```python
from build123d import *

# Parameters (mm, degrees)
SKETCH1_R           = 13.97
SKETCH1_R_2         = 1.651
BOSS_EXTRUDE1_DEPTH = 4.7625
LEG1_DEPTH          = 4.826
FILLET2_R           = 10


with BuildPart() as part:
    # Sketch1 → Boss-Extrude1 (new body)
    with BuildSketch(Plane(origin=(0, 0, 0), x_dir=(0, 0, -1), z_dir=(1, 0, 0))):
        with Locations(Location((0, 0, 0), (0, 0, 180))):
            Circle(SKETCH1_R)
        with Locations(Location((-10.16, 0, 0), (0, 0, 180))):
            Circle(SKETCH1_R_2, mode=Mode.SUBTRACT)
        with Locations(Location((0, 10.16, 0), (0, 0, 180))):
            Circle(SKETCH1_R_2, mode=Mode.SUBTRACT)
        with Locations(Location((10.16, 0, 0), (0, 0, 180))):
            Circle(SKETCH1_R_2, mode=Mode.SUBTRACT)
        with Locations(Location((0, -10.16, 0), (0, 0, 180))):
            Circle(SKETCH1_R_2, mode=Mode.SUBTRACT)
    extrude(amount=BOSS_EXTRUDE1_DEPTH)

    # Sketch2 → leg1 (add)
    with BuildSketch(Plane(origin=(4.7625, 0, 0), x_dir=(0, 0, -1), z_dir=(1, 0, 0))):
        Polygon((13.467260192, 3.714000931), (38.486260192, 3.714000931), (43.874413865, -1.674152741), (44.112587658, -5.484152741), (41.335339641, -10.038101517), (39.974157744, -4.958101517), (36.382055295, -1.365999069), (13.903055295, -1.365999069), (12.45646463, -1.365999069), (12.45646463, 3.714000931), align=None)
    extrude(amount=-LEG1_DEPTH)

    # Fillet2
    # the kernel refuses this fillet: 10 mm, written as the material it adds along each edge
    with BuildSketch(Plane(origin=(4.7625, -4.958101517, -39.974157744), x_dir=(0, 0.7071067811865493, 0.7071067811865457), z_dir=(-1, 0, 0))) as fillet2_piece_1:
        with BuildLine():
            CenterArc((FILLET2_R * 0.267949192431, -FILLET2_R), FILLET2_R, 90, 30)
            Line((-FILLET2_R * 0.232050807569, -FILLET2_R * 0.133974596216), (0, 0))
            Line((0, 0), (FILLET2_R * 0.267949192431, 0))
        make_face()
    extrude(amount=4.826)
    with BuildSketch(Plane(origin=(4.7625, -1.365999069, -36.382055295), x_dir=(0, 0, 1), z_dir=(-1, 0, 0))) as fillet2_piece_2:
        with BuildLine():
            CenterArc((FILLET2_R * 0.414213562373, -FILLET2_R), FILLET2_R, 90, 45)
            Line((-FILLET2_R * 0.292893218813, -FILLET2_R * 0.292893218813), (0, 0))
            Line((0, 0), (FILLET2_R * 0.414213562373, 0))
        make_face()
    extrude(amount=4.826)
    # the kernel refuses this fillet: 10 mm, written as the material it takes off along each edge
    with BuildSketch(Plane(origin=(15.117839059, 3.714000931, -38.486260192), x_dir=(0, 0, 1), z_dir=(-1, 0, 0))) as fillet2_2_piece_1:
        with BuildLine():
            CenterArc((FILLET2_R * 0.414213562373, -FILLET2_R), FILLET2_R, 90, 45)
            Line((-FILLET2_R * 0.292893218813, -FILLET2_R * 0.292893218813), (0, 0))
            Line((0, 0), (FILLET2_R * 0.414213562373, 0))
        make_face()
    extrude(amount=25.536678119, mode=Mode.SUBTRACT)
    with BuildSketch(Plane(origin=(14.214931239, -1.674152741, -43.874413865), x_dir=(0, 0.707106781186548, 0.707106781186547), z_dir=(-1, 0, 0))) as fillet2_2_piece_2:
        with BuildLine():
            CenterArc((FILLET2_R * 0.378097249561, -FILLET2_R), FILLET2_R, 90, 41.422934713)
            Line((-FILLET2_R * 0.283514821921, -FILLET2_R * 0.250153704503), (0, 0))
            Line((0, 0), (FILLET2_R * 0.378097249561, 0))
        make_face()
    extrude(amount=23.730862478, mode=Mode.SUBTRACT)
    with BuildSketch(Plane(origin=(12.633985106, -5.484152741, -44.112587658), x_dir=(0, -0.853758675625452, 0.5206689195585562), z_dir=(-1, 0, 0))) as fillet2_2_piece_3:
        with BuildLine():
            CenterArc((FILLET2_R * 0.314859404258, FILLET2_R), FILLET2_R, 235.045802712, 34.954197288)
            Line((-FILLET2_R * 0.258062012092, FILLET2_R * 0.180389695839), (0, 0))
            Line((0, 0), (FILLET2_R * 0.314859404258, 0))
        make_face()
    extrude(amount=20.568970213, mode=Mode.SUBTRACT)


solid = part.part
```
Design review of the part built by this model. Coordinates are the model's own, in mm. A direction names the side the tool comes from. Coordinates: 2 decimals unless noted, no trailing zeros. Loops run counter-clockwise (first coordinate to the right, second up) from the corner with the lowest first, then second, coordinate; pieces in that order, holes last. Notation, with made-up numbers: (-27, -5) -> (21, -5) arc R20 cw to (21, 5) -> close; hole circle Ø3 at (88, 45). An arc over 180 degrees is marked (long way). Answer as a JSON object with one key per item and string values.
Q1. Clearance check with flat-ended pins moving along their axes: pin 1 Ø1.4 at (x, z) = (1.5, -28.5) entering from +Y; pin 2 Ø12 at (y, z) = (-0.5, -2.5) entering from -X. State where each tip first meets the part, or that it passes through.
Answer block:
{"pin 1": "stops at y = 3.71", "pin 2": "stops at x = 0"}
Q2. Take a section at A-A on z = 0. Give the boundary of the cut face in (x, y), plus the area to 3 significant figures.
Answer block:
{"outline": "(0, -13.97) -> (4.76, -13.97) -> (4.76, -11.81) -> (0, -11.81) -> close; (0, -8.51) -> (4.76, -8.51) -> (4.76, 8.51) -> (0, 8.51) -> close; (0, 11.81) -> (4.76, 11.81) -> (4.76, 13.97) -> (0, 13.97) -> close", "area": "102 mm^2"}
Q3. Take a section at C-C on x = 2.4. Give the boundary of the cut face in (y, z).
Answer block:
{"outline": "(-10.04, -41.34) -> (-8.17, -42.47) arc R10 ccw to (-3.9, -43.89) arc R10 ccw to (0.89, -41.31) arc R10 ccw to (3.71, -34.34) -> (3.71, -13.47) arc R13.97 ccw (long way) to (-1.37, -13.9) -> (-1.37, -32.24) arc R10 cw to (-3.71, -38.67) arc R10 cw to (-7.55, -40.67) -> close; hole circle Ø3.3 at (-10.16, 0); hole circle Ø3.3 at (0, -10.16); hole circle Ø3.3 at (0, 10.16); hole circle Ø3.3 at (10.16, 0)"}
Q4. Take a section at D-D on z = -16. Give the boundary of the cut face in (x, y).
Answer block:
{"outline": "(-0.06, -1.37) -> (4.76, -1.37) -> (4.76, 3.71) -> (-0.06, 3.71) -> close"}
Q5. Tool access review of faces 4 (the flat face through (2.383, -8.81, -41.006)), 5 (the cylindrical face through (2.35, -0.07, -11.81)): name each direction out of +Z, -Z, +X, -X, +Y, -Y from which nothing blocks a thin tool from reaching the whole face with its end or side.
Answer block:
{"face 4": "+X, -X, -Y", "face 5": "+X, -X"}
Q6. The part is to be moulded in two halves that separate along Z. For faces 1 (the flat face through (-0.063, 0, -31)), 2 (the cylindrical face through (2.35, -0.07, 8.51)), 3 (the cylindrical face through (2.38, 3, -38.05)), say which applies: +Z half, -Z half, draft (parallel to the pull), parting line (faces both ways), or undercut.
Answer block:
{"face 1": "draft", "face 2": "undercut", "face 3": "-Z half"}
Q7. To check wall thickness, follow L1, parallel to Z at x = 3.45, y = -1; L2, parallel to Y at x = 2.6, z = 1; L3, parallel to Y at x = 4.45, z = 1.5. State the ranges of each line that lie inside material, in increasing order.
Answer block:
{"L1": "z = -42.75 to -11.47, -8.85 to 8.85, 11.47 to 13.93", "L2": "y = -13.93 to -11.47, -8.85 to 8.85, 11.47 to 13.93", "L3": "y = -13.89 to -10.85, -9.47 to 9.47, 10.85 to 13.89"}
Q8. Take a section at B-B on y = -2.25. Give the boundary of the cut face in (x, z), plus the area to 3 significant figures.
Answer block:
{"outline": "(-0.06, -43.37) -> (4.76, -43.37) -> (4.76, -36.35) -> (-0.06, -36.35) -> close; (0, -13.79) -> (4.76, -13.79) -> (4.76, 13.79) -> (0, 13.79) -> close", "area": "165 mm^2"}
